Could you check a few things on this model? Use its own coordinates, in mm. Face numbers are marked on the shaded views. A direction names the side the tool comes from. Give positions to 0.01 mm unless a question says otherwise; leave off trailing zeros. Write each loop counter-clockwise with the first axis right and the second up, starting at its lowest first coordinate (ties: lowest second). Pieces come first, ordered by that corner, then holes. Notation, with made-up numbers: M -12,10.5 L 27,10.5 A18 cw 27,42.5 Z; hole C 78,26 d10. An arc over 180 degrees is marked long. One line per item, written item: value.
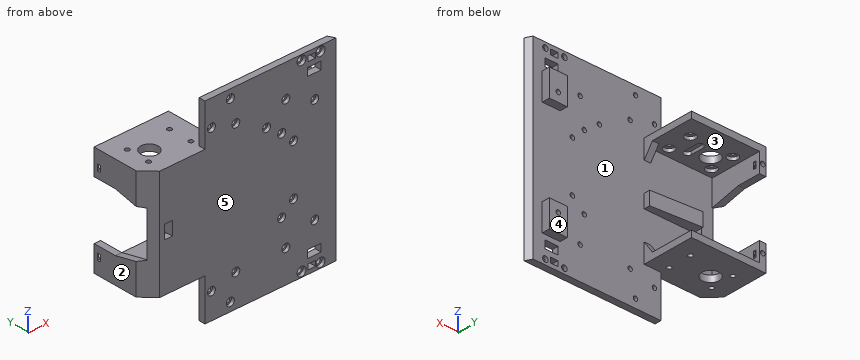
```python
from build123d import *

# Parameters (mm, degrees)
BOSS_EXTRUDE1_DEPTH = 5
BOSS_EXTRUDE2_DEPTH = 32
CUT_EXTRUDE2_DEPTH  = 5
CUT_EXTRUDE3_DEPTH  = 5
SKETCH7_R           = 6.75
SKETCH7_R_2         = 1.75
C_L_NG_C_DEPTH      = 146.27301883
SKETCH14_R          = 4
CUT_EXTRUDE8_DEPTH  = 2.5
CUT_EXTRUDE9_START  = -2.5
SKETCH15_R          = 4
CUT_EXTRUDE9_DEPTH  = 2.5
CUT_EXTRUDE15_DEPTH = 89
BOSS_EXTRUDE3_DEPTH = 8
SKETCH28_R          = 1.75
CUT_EXTRUDE16_DEPTH = 7
SKETCH29_W          = 5
SKETCH29_H          = 2.45
CUT_EXTRUDE17_DEPTH = 5
CUT_EXTRUDE18_DEPTH = 151
SKETCH30_W          = 10.5
SKETCH30_H          = 6
SKETCH30_W_2        = 6
SKETCH30_H_2        = 4
CUT_EXTRUDE19_DEPTH = 10
SKETCH31_R          = 2.15
CUT_EXTRUDE20_DEPTH = 10
SKETCH32_R          = 3.5
CUT_EXTRUDE21_DEPTH = 2.5
SKETCH34_W          = 6
SKETCH34_H          = 10.5
CUT_EXTRUDE23_DEPTH = 5
SKETCH40_R          = 1.75
CUT_EXTRUDE27_DEPTH = 5
SKETCH41_W          = 92.636025087
SKETCH41_H          = 10.5
BOSS_EXTRUDE5_DEPTH = 8
CUT_EXTRUDE28_DEPTH = 14
CUT_EXTRUDE34_DEPTH = 13.5
SKETCH49_R          = 1.75
CUT_EXTRUDE35_DEPTH = 10
SKETCH48_W          = 14
SKETCH48_H          = 21
BOSS_EXTRUDE6_DEPTH = 6
SKETCH50_R          = 1.75
CUT_EXTRUDE36_DEPTH = 19
SKETCH51_R          = 3.1
CUT_EXTRUDE37_DEPTH = 2.5


with BuildPart() as part:
    # Sketch1 → Boss-Extrude1 (new body)
    with BuildSketch(Plane(origin=(0, 0, 0), x_dir=(1, 0, 0), z_dir=(0, 1, 0))):
        Polygon((-25, 75), (-25, 42.5), (-70, 42.5), (-70, -42.5), (-25, -42.5), (-25, -75), (77, -75), (77, 75), align=None)
    extrude(amount=BOSS_EXTRUDE1_DEPTH)

    # Sketch3 → Boss-Extrude2 (add)
    with BuildSketch(Plane(origin=(0, 5, 0), x_dir=(1, 0, 0), z_dir=(0, 1, 0))):
        Polygon((-70, 17.5), (-65, 17.5), (-65, 37.5), (-17, 37.5), (-17, 27.5), (-12, 27.5), (-12, 42.5), (-70, 42.5), align=None)
        Polygon((-70, -17.5), (-70, -42.5), (-12, -42.5), (-12, -27.5), (-17, -27.5), (-17, -37.5), (-65, -37.5), (-65, -17.5), align=None)
    extrude(amount=BOSS_EXTRUDE2_DEPTH)

    # Sketch5 → Cut-Extrude2 (cut)
    with BuildSketch(Plane.ZY.offset(70)):
        Polygon((-17.5, 37), (-22.5, 37), (-22.5, 27), (-17.5, 5), align=None)
        Polygon((17.5, 5), (17.5, 37), (22.5, 37), (22.5, 27), align=None)
    extrude(amount=-CUT_EXTRUDE2_DEPTH, mode=Mode.SUBTRACT)

    # Sketch6 → Cut-Extrude3 (cut)
    with BuildSketch(Plane(origin=(-12, 0, 0), x_dir=(0, 0, -1), z_dir=(1, 0, 0))):
        Polygon((-27.5, 37), (-37.5, 37), (-37.5, 12), (-27.5, 5), align=None)
        Polygon((37.5, 12), (27.5, 5), (27.5, 37), (37.5, 37), align=None)
    extrude(amount=-CUT_EXTRUDE3_DEPTH, mode=Mode.SUBTRACT)

    # Sketch7 → c l_ _ng c (cut, through all)
    with BuildSketch(Plane(origin=(0, 0, -42.5), x_dir=(-1, 0, 0), z_dir=(0, 0, -1))):
        with Locations((49, 21)):
            Circle(SKETCH7_R)
        with Locations((25, 30)):
            Circle(SKETCH7_R_2)
        with Locations((25, 12)):
            Circle(SKETCH7_R_2)
        with Locations((58, 30)):
            Circle(SKETCH7_R_2)
        with Locations((58, 12)):
            Circle(SKETCH7_R_2)
    extrude(amount=-C_L_NG_C_DEPTH, mode=Mode.SUBTRACT)

    # Sketch14 → Cut-Extrude8 (cut)
    with BuildSketch(Plane(origin=(0, 0, 37.5), x_dir=(-1, 0, 0), z_dir=(0, 0, -1))):
        with Locations((58, 30)):
            Circle(SKETCH14_R)
        with Locations((25, 30)):
            Circle(SKETCH14_R)
        with Locations((25, 12)):
            Circle(SKETCH14_R)
        with Locations((58, 12)):
            Circle(SKETCH14_R)
        with BuildLine():
            Line((38.8, 26.25), (38.8, 15.75))
            ThreePointArc((38.8, 15.75), (36, 12.95), (33.2, 15.75))
            Line((33.2, 15.75), (33.2, 26.25))
            ThreePointArc((33.2, 26.25), (36, 29.05), (38.8, 26.25))
        make_face()
    extrude(amount=-CUT_EXTRUDE8_DEPTH, mode=Mode.SUBTRACT)

    # Sketch15 → Cut-Extrude9 (cut)
    with BuildSketch(Plane.XY.offset(-37.5).offset(CUT_EXTRUDE9_START)):
        with Locations(Location((-25, 30, 0), (0, 0, 180))):
            Circle(SKETCH15_R)
        with Locations(Location((-25, 12, 0), (0, 0, 180))):
            Circle(SKETCH15_R)
        with Locations(Location((-58, 12, 0), (0, 0, 180))):
            Circle(SKETCH15_R)
        with Locations(Location((-58, 30, 0), (0, 0, 180))):
            Circle(SKETCH15_R)
        with BuildLine():
            Line((-33.2, 26.25), (-33.2, 15.75))
            ThreePointArc((-33.2, 15.75), (-36, 12.95), (-38.8, 15.75))
            Line((-38.8, 15.75), (-38.8, 26.25))
            ThreePointArc((-38.8, 26.25), (-36, 29.05), (-33.2, 26.25))
        make_face()
    extrude(amount=CUT_EXTRUDE9_DEPTH, mode=Mode.SUBTRACT)

    # Sketch25 → Cut-Extrude15 (cut)
    with BuildSketch(Plane.XY.offset(42.5)):
        Polygon((-70, 9.5), (-70, 0), (-60.5, 0), align=None)
    extrude(amount=-CUT_EXTRUDE15_DEPTH, mode=Mode.SUBTRACT)

    # Sketch27 → Boss-Extrude3 (add)
    with BuildSketch(Plane(origin=(0, 37, 0), x_dir=(1, 0, 0), z_dir=(0, 1, 0))):
        Polygon((-12, 42.5), (-70, 42.5), (-70, 22.5), (-65, 22.5), (-65, 37.5), (-12, 37.5), align=None)
        Polygon((-12, -37.5), (-12, -42.5), (-70, -42.5), (-70, -22.5), (-65, -22.5), (-65, -37.5), align=None)
    extrude(amount=BOSS_EXTRUDE3_DEPTH)

    # Sketch28 → Cut-Extrude16 (cut)
    with BuildSketch(Plane(origin=(0, 45, 0), x_dir=(1, 0, 0), z_dir=(0, 1, 0))):
        with Locations(Location((-67.5, -30, 0), (0, 0, 270))):
            Circle(SKETCH28_R)
        with Locations(Location((-67.5, 30, 0), (0, 0, 90))):
            Circle(SKETCH28_R)
    extrude(amount=-CUT_EXTRUDE16_DEPTH, mode=Mode.SUBTRACT)

    # Sketch29 → Cut-Extrude17 (cut)
    with BuildSketch(Plane.ZY.offset(70)):
        with Locations((-30, 41)):
            Rectangle(SKETCH29_W, SKETCH29_H)
        with Locations((30, 41)):
            Rectangle(SKETCH29_W, SKETCH29_H)
    extrude(amount=-CUT_EXTRUDE17_DEPTH, mode=Mode.SUBTRACT)

    # Sketch26 → Cut-Extrude18 (cut)
    with BuildSketch(Plane.XY.offset(75)):
        Polygon((74.668461709, 5), (77, 0), (77, 5), align=None)
    extrude(amount=-CUT_EXTRUDE18_DEPTH, mode=Mode.SUBTRACT)

    # Sketch30 → Cut-Extrude19 (cut)
    with BuildSketch(Plane(origin=(0, 0, 0), x_dir=(-1, 0, 0), z_dir=(0, -1, 0))):
        with Locations((-60.25, 61.25)):
            Rectangle(SKETCH30_W, SKETCH30_H)
        with Locations((-60.25, -61.25)):
            Rectangle(SKETCH30_W, SKETCH30_H)
        with Locations((-58.17, -70)):
            Rectangle(SKETCH30_W_2, SKETCH30_H_2)
        with Locations((-58.17, 70)):
            Rectangle(SKETCH30_W_2, SKETCH30_H_2)
    extrude(amount=-CUT_EXTRUDE19_DEPTH, mode=Mode.SUBTRACT)

    # Sketch31 → Cut-Extrude20 (cut)
    with BuildSketch(Plane(origin=(0, 0, 0), x_dir=(-1, 0, 0), z_dir=(0, -1, 0))):
        with Locations(Location((-65, -71, 0), (0, 0, 90))):
            Circle(SKETCH31_R)
        with Locations(Location((-50.22, -71, 0), (0, 0, 90))):
            Circle(SKETCH31_R)
        with Locations(Location((-50.22, 71, 0), (0, 0, 90))):
            Circle(SKETCH31_R)
        with Locations(Location((-65, 71, 0), (0, 0, 90))):
            Circle(SKETCH31_R)
    extrude(amount=-CUT_EXTRUDE20_DEPTH, mode=Mode.SUBTRACT)

    # Sketch32 → Cut-Extrude21 (cut)
    with BuildSketch(Plane(origin=(0, 0, 0), x_dir=(-1, 0, 0), z_dir=(0, -1, 0))):
        with Locations(Location((-65, -71, 0), (0, 0, 90))):
            Circle(SKETCH32_R)
        with Locations(Location((-50.22, -71, 0), (0, 0, 90))):
            Circle(SKETCH32_R)
        with Locations(Location((-50.22, 71, 0), (0, 0, 270))):
            Circle(SKETCH32_R)
        with Locations(Location((-65, 71, 0), (0, 0, 270))):
            Circle(SKETCH32_R)
    extrude(amount=-CUT_EXTRUDE21_DEPTH, mode=Mode.SUBTRACT)

    # Sketch34 → Cut-Extrude23 (cut)
    with BuildSketch(Plane(origin=(0, 0, 0), x_dir=(-1, 0, 0), z_dir=(0, -1, 0))):
        with Locations((53.546244223, 0)):
            Rectangle(SKETCH34_W, SKETCH34_H)
    extrude(amount=-CUT_EXTRUDE23_DEPTH, mode=Mode.SUBTRACT)

    # Sketch40 → Cut-Extrude27 (cut)
    with BuildSketch(Plane(origin=(0, 0, 0), x_dir=(-1, 0, 0), z_dir=(0, -1, 0))):
        with Locations(Location((-38, -50, 0), (0, 0, 90))):
            Circle(SKETCH40_R)
        with Locations(Location((-34.75, -28.4, 0), (0, 0, 90))):
            Circle(SKETCH40_R)
        with Locations(Location((-44, -19.5, 0), (0, 0, 90))):
            Circle(SKETCH40_R)
        with Locations(Location((20, -55, 0), (0, 0, 90))):
            Circle(SKETCH40_R)
        with Locations(Location((5.25, -68.4, 0), (0, 0, 90))):
            Circle(SKETCH40_R)
        with Locations(Location((1, -50, 0), (0, 0, 90))):
            Circle(SKETCH40_R)
        with Locations(Location((1, 50, 0), (0, 0, 270))):
            Circle(SKETCH40_R)
        with Locations(Location((5.25, 68.4, 0), (0, 0, 270))):
            Circle(SKETCH40_R)
        with Locations(Location((20, 55, 0), (0, 0, 270))):
            Circle(SKETCH40_R)
        with Locations(Location((-44, 19.5, 0), (0, 0, 270))):
            Circle(SKETCH40_R)
        with Locations(Location((-34.75, 28.4, 0), (0, 0, 270))):
            Circle(SKETCH40_R)
        with Locations(Location((-38, 50, 0), (0, 0, 270))):
            Circle(SKETCH40_R)
    extrude(amount=-CUT_EXTRUDE27_DEPTH, mode=Mode.SUBTRACT)

    # Sketch41 → Boss-Extrude5 (add)
    with BuildSketch(Plane(origin=(0, 5, 0), x_dir=(1, 0, 0), z_dir=(0, 1, 0))):
        with Locations((-4.228231679, 0)):
            Rectangle(SKETCH41_W, SKETCH41_H)
    extrude(amount=BOSS_EXTRUDE5_DEPTH)

    # Sketch42 → Cut-Extrude28 (cut)
    with BuildSketch(Plane.XY.offset(5.25)):
        Polygon((42.089780864, 5), (42.089780864, 13), (-50.546244223, 13), align=None)
    extrude(amount=-CUT_EXTRUDE28_DEPTH, mode=Mode.SUBTRACT)

    # Sketch47 → Cut-Extrude34 (cut)
    with BuildSketch(Plane.XY.offset(5.25)):
        Polygon((-12, 9.671165958), (-12, 5), (42.089780864, 5), align=None)
    extrude(amount=-CUT_EXTRUDE34_DEPTH, mode=Mode.SUBTRACT)

    # Sketch49 → Cut-Extrude35 (cut)
    with BuildSketch(Plane(origin=(0, 0, 0), x_dir=(-1, 0, 0), z_dir=(0, -1, 0))):
        with Locations(Location((-23, -37, 0), (0, 0, 90))):
            Circle(SKETCH49_R)
    extrude(amount=-CUT_EXTRUDE35_DEPTH, mode=Mode.SUBTRACT)

    # Sketch48 → Boss-Extrude6 (add)
    with BuildSketch(Plane(origin=(0, 5, 0), x_dir=(1, 0, 0), z_dir=(0, 1, 0))):
        with Locations((60.5, 44)):
            Rectangle(SKETCH48_W, SKETCH48_H)
        with Locations((60.5, -44)):
            Rectangle(SKETCH48_W, SKETCH48_H)
    extrude(amount=BOSS_EXTRUDE6_DEPTH)

    # Sketch50 → Cut-Extrude36 (cut)
    with BuildSketch(Plane(origin=(0, 0, 0), x_dir=(-1, 0, 0), z_dir=(0, -1, 0))):
        with Locations(Location((-60.5, -40.5, 0), (0, 0, 90))):
            Circle(SKETCH50_R)
        with Locations(Location((-60.5, 40.5, 0), (0, 0, 270))):
            Circle(SKETCH50_R)
    extrude(amount=-CUT_EXTRUDE36_DEPTH, mode=Mode.SUBTRACT)

    # Sketch51 → Cut-Extrude37 (cut)
    with BuildSketch(Plane(origin=(0, 0, 0), x_dir=(-1, 0, 0), z_dir=(0, -1, 0))):
        with Locations(Location((-60.5, -40.5, 0), (0, 0, 90))):
            Circle(SKETCH51_R)
        with Locations(Location((-44, -19.5, 0), (0, 0, 90))):
            Circle(SKETCH51_R)
        with Locations(Location((-34.75, -28.4, 0), (0, 0, 90))):
            Circle(SKETCH51_R)
        with Locations(Location((-38, -50, 0), (0, 0, 90))):
            Circle(SKETCH51_R)
        with Locations(Location((-23, -37, 0), (0, 0, 90))):
            Circle(SKETCH51_R)
        with Locations(Location((1, -50, 0), (0, 0, 90))):
            Circle(SKETCH51_R)
        with Locations(Location((5.25, -68.4, 0), (0, 0, 90))):
            Circle(SKETCH51_R)
        with Locations(Location((20, -55, 0), (0, 0, 90))):
            Circle(SKETCH51_R)
        with Locations(Location((20, 55, 0), (0, 0, 270))):
            Circle(SKETCH51_R)
        with Locations(Location((5.25, 68.4, 0), (0, 0, 270))):
            Circle(SKETCH51_R)
        with Locations(Location((1, 50, 0), (0, 0, 270))):
            Circle(SKETCH51_R)
        with Locations(Location((-38, 50, 0), (0, 0, 270))):
            Circle(SKETCH51_R)
        with Locations(Location((-34.75, 28.4, 0), (0, 0, 270))):
            Circle(SKETCH51_R)
        with Locations(Location((-44, 19.5, 0), (0, 0, 270))):
            Circle(SKETCH51_R)
        with Locations(Location((-60.5, 40.5, 0), (0, 0, 270))):
            Circle(SKETCH51_R)
    extrude(amount=-CUT_EXTRUDE37_DEPTH, mode=Mode.SUBTRACT)


solid = part.part
```
1) Please list where these lines run through material, in increasing order: L1, parallel to X at y = 30, z = -39; L2, parallel to Y at x = -25, z = 38.05; L3, parallel to Y at x = -49, z = 38. Write a range as from..to.
Outcome:
L1: x = -70..-62, -54..-29, -21..-12
L2: y = 0..8, 16..26, 34..45
L3: y = 0..14.25, 27.75..45
2) If we section it at B-B, the plane y = 23: Write out the boundary of the cut face in (x, z).
Outcome:
outline: M -70,-42.5 L -55.45,-42.5 L -55.45,-37.5 L -65,-37.5 L -65,-21.59 L -70,-21.59 Z; M -70,21.59 L -65,21.59 L -65,37.5 L -55.45,37.5 L -55.45,42.5 L -70,42.5 Z; M -42.55,-42.5 L -12,-42.5 L -12,-37.5 L -33.2,-37.5 L -33.2,-40 L -38.8,-40 L -38.8,-37.5 L -42.55,-37.5 Z; M -42.55,37.5 L -38.8,37.5 L -38.8,40 L -33.2,40 L -33.2,37.5 L -12,37.5 L -12,42.5 L -42.55,42.5 Z
3) If we section it at D-D, the plane x = 11: Write out the boundary of the cut face in (y, z).
Outcome:
outline: M 0,-75 L 5,-75 L 5,75 L 0,75 Z
4) If we section it at C-C, the plane x = -36: Write out the boundary of the cut face in (y, z).
Outcome:
outline: M 0,-42.5 L 45,-42.5 L 45,-37.5 L 29.05,-37.5 L 29.05,-40 L 12.95,-40 L 12.95,-37.5 L 5,-37.5 L 5,-5.25 L 11.74,-5.25 L 11.74,5.25 L 5,5.25 L 5,37.5 L 12.95,37.5 L 12.95,40 L 29.05,40 L 29.05,37.5 L 45,37.5 L 45,42.5 L 0,42.5 Z
5) I'm going to push flat-ended pins straight in: pin 1 (2 mm diameter, centred on x = 53.5, z = 28, fed in from -Y); pin 2 (3 mm diameter, centred on y = 4.5, z = -2, fed in from -X); pin 3 (2.5 mm diameter, centred on x = -68.5, z = 30.5, fed in from -Y); pin 4 (6 mm diameter, centred on y = 14.5, z = -2, fed in from -X). Where does each tip first touch, or does it pass through?
Outcome:
pin 1: stops at y = 0
pin 2: stops at x = -65.5
pin 3: stops at y = 6.75
pin 4: stops at x = -50.55
6) We'd pull the mould along Z, two halves only. Please class the marked faces 1 and 2: pulls with the +Z half, pulls with the -Z half, needs draft (parallel to the pull), parting line crosses it, or undercut.
Outcome:
face 1: undercut
face 2: needs draft
7) If we section it at A-A, the plane z = 1: Write out the boundary of the cut face in (x, y), then the cut area to 3 significant figures.
Outcome:
outline: M -65.5,5 L -60.5,0 L -56.55,0 L -56.55,5 Z; M -50.55,0 L 77,0 L 74.67,5 L -12,5 L -12,9.67 L -50.55,13 Z
area: 908 mm^2
8) On a 3-axis mill with a long thin cutter (end or side, diameter ignored), from which of +Z, -Z, +X, -X, +Y, -Y can I reach the whole of each face in a straight line? I mean the marked faces 3, 4 and 5. Say none if no direction works.
Outcome:
face 3: +Y
face 4: +Z, -Z, +X, +Y
face 5: +Z, -Z, +X, -X, -Y
